from build123d import *

# Parameters (mm, degrees)
F1_DEPTH = 38.1
F2_DEPTH = 25.4
F3_DEPTH = 12.7
F4_DEPTH = 12.7


with BuildPart() as f1:
    # F0 (on Front) → F1 (new body)
    with BuildSketch(Plane.XZ):
        Polygon((0, 6.35), (0, 0), (25.4, 0), (25.4, 6.35), (14.816667, 6.35), align=None)
    extrude(amount=F1_DEPTH)

    # F0 (on Front) → F2 (join)
    with BuildSketch(Plane.XZ):
        Polygon((0, 19.446875), (0, 6.35), (14.816667, 6.35), (14.816667, 14.2875), (7.9375, 19.446875), align=None)
    extrude(amount=F2_DEPTH)

    # F0 (on Front) → F3 (join)
    with BuildSketch(Plane.XZ):
        Polygon((0, 25.4), (0, 19.446875), (7.9375, 19.446875), align=None)
    extrude(amount=F3_DEPTH)

    # F0 (on Front) → F4 (join)
    with BuildSketch(Plane.XZ):
        Polygon((14.816667, 14.2875), (14.816667, 6.35), (25.4, 6.35), align=None)
    extrude(amount=F4_DEPTH)


solid = f1.part
The model under review builds one solid part; all positions refer to its coordinate system, in mm. A direction names the side the tool comes from. Give positions to 0.01 mm unless a question says otherwise; leave off trailing zeros. Order: outer loops, then holes, each group sorted by start corner. A loop starts at its lowest first (then second) coordinate and runs counter-clockwise, first axis right, second up. Notation, with made-up numbers: M 1,28 L 60,28 A21 ccw 60,47 Z; hole C 13,37.25 d9. An arc over 180 degrees is marked long. One line per question, with ' | ' between items. Start each with the question number.
1) Consider section C-C, the plane x = 7. Give the boundary of the cut face in (y, z).
2) Consider section D-D, the plane x = 13. Give the boundary of the cut face in (y, z).
3) Consider section A-A, the plane y = -18.5. Give the boundary of the cut face in (x, z), then the cut area to 3 significant figures.
4) Consider section B-B, the plane z = 10.25. Give the boundary of the cut face in (x, y), then the cut area to 3 significant figures.
5) Wall thickness on L1, parallel to Z at x = 3, y = -36; L2, parallel to Y at x = 7.5, z = 19; L3, parallel to X at y = -9, z = 18.5: over which ranges is each line inside the solid? List them lowest first. Write a range as from..to.
6) For faces 1 (the face through (2, -12.7, 21)), 2 (the face through (18, -12.7, 9)), 3 (the face through (13, -19, 0)), list the 3-axis set-ups (+Z, -Z, +X, -X, +Y, -Y) from which the entire face can be reached by the end or side of a thin tool; tool diameter is ignored.
7) Clearance check with flat-ended pins moving along their axes: P1, Ø8.5, axis at x = 2, y = -17, coming from the +Z side; P2, Ø5, axis at x = 4, z = 22, coming from the -Y side; P3, Ø4, axis at y = -22, z = 8.5, coming from the +X side. State where each tip first meets the part, or that it passes through.
Found:
1) outline: M -38.1,0 L 0,0 L 0,20.15 L -12.7,20.15 L -12.7,19.45 L -25.4,19.45 L -25.4,6.35 L -38.1,6.35 Z
2) outline: M -38.1,0 L 0,0 L 0,15.65 L -25.4,15.65 L -25.4,6.35 L -38.1,6.35 Z
3) outline: M 0,0 L 25.4,0 L 25.4,6.35 L 14.82,6.35 L 14.82,14.29 L 7.94,19.45 L 0,19.45 Z | area: 338 mm²
4) outline: M 0,-25.4 L 14.82,-25.4 L 14.82,-12.7 L 20.2,-12.7 L 20.2,0 L 0,0 Z | area: 445 mm²
5) L1: z = 0..6.35 | L2: y = -25.4..0 | L3: x = 0..9.2
6) face 1: +Z, +X, -X, -Y | face 2: +Z, +X, -Y | face 3: -Z, +X, -X, +Y, -Y
7) P1: stops at z = 19.45 | P2: stops at y = -12.7 | P3: stops at x = 14.82
